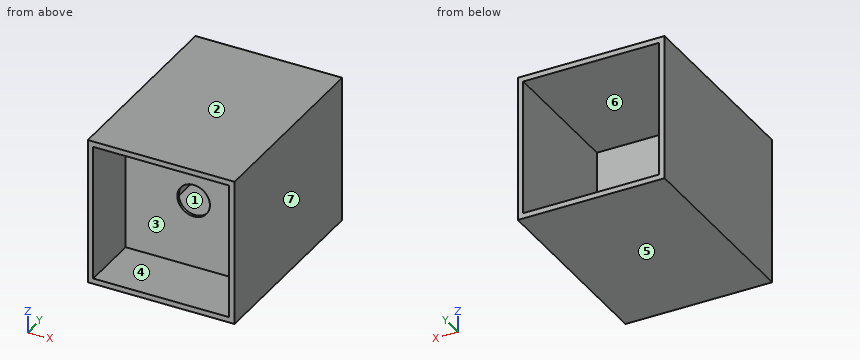
```python
from build123d import *

# Parameters (mm, degrees)
SKETCH1_W           = 54
SKETCH1_H           = 54
SKETCH1_W_2         = 50
SKETCH1_H_2         = 50
BOSS_EXTRUDE1_DEPTH = 22
SKETCH2_W           = 54
SKETCH2_H           = 54
BOSS_EXTRUDE2_DEPTH = 1
SKETCH3_R           = 6
CUT_EXTRUDE1_DEPTH  = 24
SKETCH4_W           = 2
SKETCH4_H           = 50
SKETCH4_H_2         = 2
SKETCH4_W_2         = 50
BOSS_EXTRUDE3_DEPTH = 50


with BuildPart() as part:
    # Sketch1 → Boss-Extrude1 (new body)
    with BuildSketch(Plane(origin=(0, 0, 0), x_dir=(1, 0, 0), z_dir=(0, 1, 0))):
        Rectangle(SKETCH1_W, SKETCH1_H)
        Rectangle(SKETCH1_W_2, SKETCH1_H_2, mode=Mode.SUBTRACT)
    extrude(amount=BOSS_EXTRUDE1_DEPTH)

    # Sketch2 → Boss-Extrude2 (add)
    with BuildSketch(Plane(origin=(0, 22, 0), x_dir=(1, 0, 0), z_dir=(0, 1, 0))):
        Rectangle(SKETCH2_W, SKETCH2_H)
    extrude(amount=BOSS_EXTRUDE2_DEPTH)

    # Sketch3 → Cut-Extrude1 (cut, through all)
    with BuildSketch(Plane(origin=(0, 23, 0), x_dir=(1, 0, 0), z_dir=(0, 1, 0))):
        Circle(SKETCH3_R)
    extrude(amount=-CUT_EXTRUDE1_DEPTH, mode=Mode.SUBTRACT)

    # Sketch4 → Boss-Extrude3 (add)
    with BuildSketch(Plane(origin=(0, 23, 0), x_dir=(1, 0, 0), z_dir=(0, 1, 0))):
        with Locations((-26, 0)):
            Rectangle(SKETCH4_W, SKETCH4_H)
        with Locations((-26, -26)):
            Rectangle(SKETCH4_W, SKETCH4_H_2)
        with Locations((0, -26)):
            Rectangle(SKETCH4_W_2, SKETCH4_H_2)
        with Locations((26, -26)):
            Rectangle(SKETCH4_W, SKETCH4_H_2)
        with Locations((26, 0)):
            Rectangle(SKETCH4_W, SKETCH4_H)
        with Locations((26, 26)):
            Rectangle(SKETCH4_W, SKETCH4_H_2)
        with Locations((0, 26)):
            Rectangle(SKETCH4_W_2, SKETCH4_H_2)
        with Locations((-26, 26)):
            Rectangle(SKETCH4_W, SKETCH4_H_2)
    extrude(amount=BOSS_EXTRUDE3_DEPTH)


solid = part.part
```
Geometry check sheet. Reference: the model listing, model coordinates, mm. Face numbers are marked on the shaded views. A direction names the side the tool comes from. Coordinates: 2 decimals unless noted, no trailing zeros. Order: outer loops, then holes, each group sorted by start corner. A loop starts at its lowest first (then second) coordinate and runs counter-clockwise, first axis right, second up. Notation, with made-up numbers: M 36.25,-27 L 50.25,-27 A23 ccw 50.25,3 Z; hole C -37.75,85 d2. An arc over 180 degrees is marked long. One line per question, with ' | ' between items. Start each with the question number.
Item 1: Material ranges on L1, parallel to X at y = 22.65, z = 0; L2, parallel to X at y = 32, z = -4.5, recorded low to high. Write a range as [from, to].
Item 2: Cross-section at B-B on y = 59.5. Enter the section's corners in (x, z), then the cut area to 3 significant figures.
Item 3: Cross-section at C-C on z = 0. Enter the section's corners in (x, y).
Item 4: Draft check along Z on the marked faces 4, 5, 6 and 7. Enter one of: pulls with the +Z half, pulls with the -Z half, needs draft (parallel to the pull), parting line crosses it, or undercut.
Item 5: Cross-section at D-D on x = 10. Enter the section's corners in (y, z).
Item 6: Gauge pin test, flat ends, axial feed: pin 1 (6 mm diameter, centred on x = -16.5, z = 14, fed in from -Y); pin 2 (8 mm diameter, centred on x = 10, z = -8, fed in from +Y). Record the tip position at first contact, or that the pin passes through.
Item 7: Cross-section at A-A on x = 0. Enter the section's corners in (y, z), then the cut area to 3 significant figures.
Item 8: Set-up check for the marked faces 1, 2 and 3: record each of +Z, -Z, +X, -X, +Y, -Y from which the full face is reachable in a straight line by a thin tool's end or side.
Findings:
1) L1: x = [-27, -6], [6, 27] | L2: x = [-27, -25], [25, 27]
2) outline: M -27,-27 L 27,-27 L 27,27 L -27,27 Z; hole M -25,-25 L 25,-25 L 25,25 L -25,25 Z | area: 416 mm²
3) outline: M -27,0 L -25,0 L -25,22 L -6,22 L -6,23 L -25,23 L -25,73 L -27,73 Z; M 6,22 L 25,22 L 25,0 L 27,0 L 27,73 L 25,73 L 25,23 L 6,23 Z
4) face 4: undercut | face 5: pulls with the -Z half | face 6: undercut | face 7: needs draft
5) outline: M 0,-27 L 73,-27 L 73,-25 L 23,-25 L 23,25 L 73,25 L 73,27 L 0,27 L 0,25 L 22,25 L 22,-25 L 0,-25 Z
6) pin 1: stops at y = 22 | pin 2: stops at y = 23
7) outline: M 0,-27 L 73,-27 L 73,-25 L 23,-25 L 23,-6 L 22,-6 L 22,-25 L 0,-25 Z; M 0,25 L 22,25 L 22,6 L 23,6 L 23,25 L 73,25 L 73,27 L 0,27 Z | area: 330 mm²
8) face 1: +Y | face 2: +Z, +X, -X, +Y, -Y | face 3: -Y
